Autodesk Fusion 360 part; units mm, degrees
sketch "Sketch1" plane through (0, 0, 0) normal (0, 1, 0) x (1, 0, 0)
  arc A0 (-1.5, 2.1237) -> (1.5, 2.1237) centre (0, 0) ccw
  line L0 (-1.5, 2.1237) -> (1.5, 2.1237)
  arc A1 (1.75, -3.4853) -> (1.75, 3.4853) centre (0, 0) ccw
  arc A2 (-1.75, 3.4853) -> (-1.75, -3.4853) centre (0, 0) ccw
  line L1 (-1.75, 3.4853) -> (1.75, 3.4853)
  line L2 (1.75, -3.4853) -> (-1.75, -3.4853)
  dimension "d1" = 2.6
  dimension "d2" = 3
  dimension "d3" = 3.9
  dimension "d4" = 3.9
  dimension "d5" = 3.5
  dimension "d6" = 3.5
extrude "Extrude1" add sketch "Sketch1" along normal blind 3.5
Check sheet for the modelled part. Datum: model origin and axes. Units: mm. A direction names the side the tool comes from. Round coordinates to 2 decimals unless told otherwise and drop trailing zeros. Order: outer loops, then holes, each group sorted by start corner. A loop starts at its lowest first (then second) coordinate and runs counter-clockwise, first axis right, second up.
1) Section check C-C (y = 3.15). Record the boundary of the cut face in (x, z).
2) Scan lines: line 1 (Z direction, x = 0, y = 2.2); line 2 (Z direction, x = 2.25, y = 2.6); line 3 (X direction, y = 3.05, z = -0.25). Record each from-to range of solid material in increasing order.
3) Section check D-D (z = 3.25). Record the boundary of the cut face in (x, y).
4) Section check A-A (z = 0). Record the boundary of the cut face in (x, y).
5) Go/stop test with a flat-tipped pin: pin 1 Ø3 at (x, z) = (0, 0) entering from +Y. Record where the tip stops, or that it passes through.
6) Mould release check, pull along Z, two halves, no side actions. Record for faces 1 (the flat face through (0, 2, 3.485)), 2 (the flat face through (-0.1, 3.5, -2.4)), 3 (the cylindrical face through (0.1, 1.7, 2.6)): +Z half, -Z half, draft (parallel to the pull), parting line (faces both ways), or undercut.
7) Section check B-B (x = 0). Record the boundary of the cut face in (y, z).
8) Tool access check on faces 4 (the flat face through (0, 2, -3.485)), 5 (the flat face through (0, 2, -2.124)). Record the directions out of +Z, -Z, +X, -X, +Y, -Y that give a thin tool (end or side, any length) a straight path to the whole face; none if there is none.
Result:
1. outline: (-1.75, -3.49) - (1.75, -3.49) arc R3.9 ccw to (1.75, 3.49) - (-1.75, 3.49) arc R3.9 ccw to start; hole (-1.5, -2.12) - (1.5, -2.12) arc R2.6 ccw (long way) to start
2. line 1: z = -3.49 to -2.12, 2.6 to 3.49
2. line 2: z = -3.19 to -1.3, 1.3 to 3.19
2. line 3: x = -3.89 to -2.59, 2.59 to 3.89
3. outline: (-2.16, 0) - (2.16, 0) - (2.16, 3.5) - (-2.16, 3.5) - close
4. outline: (-3.9, 0) - (-2.6, 0) - (-2.6, 3.5) - (-3.9, 3.5) - close; (2.6, 0) - (3.9, 0) - (3.9, 3.5) - (2.6, 3.5) - close
5. pin 1: passes through
6. face 1: +Z half
6. face 2: draft
6. face 3: undercut
7. outline: (0, -3.49) - (3.5, -3.49) - (3.5, -2.12) - (0, -2.12) - close; (0, 2.6) - (3.5, 2.6) - (3.5, 3.49) - (0, 3.49) - close
8. face 4: -Z, +X, -X, +Y, -Y
8. face 5: +Y, -Y
